Build history of the part. All positions in model axes, mm. A direction names the side the tool comes from. Round coordinates to 2 decimals unless told otherwise and drop trailing zeros. Write each loop counter-clockwise with the first axis right and the second up, starting at its lowest first coordinate (ties: lowest second). Pieces come first, ordered by that corner, then holes.
Item 1: Band-saw the part on A-A, the plane y = 21.5. Write the cut outline in (x, z), then the cut area to 3 significant figures.
Item 2: Wall check: probe 1 along Y at (x, z) = (0.45, -0.3); probe 2 along Y at (x, z) = (-0.8, 1.9); probe 3 along Z at (x, y) = (-0.1, 39). Give the ranges that are in metal, low to high.
Item 3: Drop flat-ended pins along their axis: pin 1 Ø1.5 at (x, y) = (1, 15) entering from -Z; pin 2 Ø2 at (x, y) = (-2, 5.5) entering from +Z; pin 3 Ø2 at (y, z) = (8.5, -1) entering from -X. Give the stop position or say it passes through.
Item 4: 3-axis set-ups, long thin cutter, end or side, ignore diameter. For faces 1 (the flat face through (1.3, 0, -1.3)), 2 (the flat face through (0, -2, 0)): which of +Z, -Z, +X, -X, +Y, -Y reach the whole face in a straight line?
Item 5: Band-saw the part on B-B, the plane z = -2.3. Write the cut outline in (x, y).
```python
from build123d import *

# Parameters (mm, degrees)
SKETCH2_R           = 1.5
BOSS_EXTRUDE1_DEPTH = 5
SKETCH3_R           = 0.5
BOSS_EXTRUDE2_DEPTH = 60
SKETCH4_R           = 3
BOSS_EXTRUDE3_DEPTH = 2


with BuildPart() as part:
    # Sketch2 → Boss-Extrude1 (new body)
    with BuildSketch(Plane(origin=(0, 0, 0), x_dir=(1, 0, 0), z_dir=(0, 1, 0))):
        Circle(SKETCH2_R)
    extrude(amount=BOSS_EXTRUDE1_DEPTH)

    # Sketch3 → Boss-Extrude2 (add)
    with BuildSketch(Plane(origin=(0, 5, 0), x_dir=(1, 0, 0), z_dir=(0, 1, 0))):
        Circle(SKETCH3_R)
    extrude(amount=BOSS_EXTRUDE2_DEPTH)

    # Sketch4 → Boss-Extrude3 (add)
    with BuildSketch(Plane.XZ):
        Circle(SKETCH4_R)
    extrude(amount=BOSS_EXTRUDE3_DEPTH)


solid = part.part
```
Results:
1. outline: circle Ø1 at (0, 0)
1. area: 0.785 mm2
2. probe 1: y = -2 to 5
2. probe 2: y = -2 to 0
2. probe 3: z = -0.49 to 0.49
3. pin 1: stops at z = -0.43
3. pin 2: stops at z = 0.98
3. pin 3: stops at x = -0.5
4. face 1: +Y
4. face 2: +Z, -Z, +X, -X, -Y
5. outline: (-1.93, -2) - (1.93, -2) - (1.93, 0) - (-1.93, 0) - close
